Autodesk Inventor part; units mm, degrees
ref_plane "YZ Plane" through (0, 0, 0) normal (1, 0, 0) x (0, 1, 0)
ref_plane "XZ Plane" through (0, 0, 0) normal (0, 1, 0) x (-1, 0, 0)
ref_plane "XY Plane" through (0, 0, 0) normal (0, 0, 1) x (1, 0, 0)
sketch "Sketch1" plane through (0, 0, 0) normal (0, 0, 1) x (1, 0, 0)
  line L0 (-75, -60) -> (75, -60)
  line L1 (75, -60) -> (75, 60)
  line L2 (75, 60) -> (-75, 60)
  line L3 (-75, 60) -> (-75, -60)
  line L4 (-75, -60) -> (75, 60) construction
  line L5 (75, -60) -> (-75, 60) construction
  line L6 (-70, -55) -> (70, -55) construction
  line L7 (70, -55) -> (70, 55) construction
  line L8 (70, 55) -> (-70, 55) construction
  line L9 (-70, 55) -> (-70, -55) construction
  circle A0 centre (-48, 0) radius 15
  circle A1 centre (-55, 55) radius 1.6
  circle A2 centre (-18.3333, 55) radius 1.6
  circle A3 centre (18.3333, 55) radius 1.6
  circle A4 centre (55, 55) radius 1.6
  circle A5 centre (-55.8297, -55) radius 1.6
  circle A6 centre (-19.1631, -55) radius 1.6
  circle A7 centre (17.5036, -55) radius 1.6
  circle A8 centre (54.1703, -55) radius 1.6
  circle A9 centre (-65.3, 4) radius 1.25
  circle A10 centre (-30.7, 4) radius 1.25
  circle A11 centre (-65.3, -40) radius 1.25
  circle A12 centre (-30.7, -40) radius 1.25
  circle A13 centre (48, 0) radius 15
  circle A14 centre (30.7, 4) radius 1.25
  circle A15 centre (65.3, 4) radius 1.25
  circle A16 centre (30.7, -40) radius 1.25
  circle A17 centre (65.3, -40) radius 1.25
  circle A18 centre (0, -25) radius 15
  circle A19 centre (17.3, -29) radius 1.25
  circle A20 centre (-17.3, -29) radius 1.25
  circle A21 centre (17.3, 15) radius 1.25
  circle A22 centre (-17.3, 15) radius 1.25
  line L10 (-62.5, 19) -> (-62.5, 31) construction
  line L11 (-59.5, 19) -> (-59.5, 31) construction
  line L12 (-65.5, 31) -> (-65.5, 19) construction
  arc A23 (-65.5, 19) -> (-59.5, 19) centre (-62.5, 19) ccw construction
  arc A24 (-59.5, 31) -> (-65.5, 31) centre (-62.5, 31) ccw construction
  line L13 (-58, 31) -> (-58, 19)
  arc A25 (-67, 19) -> (-58, 19) centre (-62.5, 19) ccw
  line L14 (-67, 19) -> (-67, 31)
  arc A26 (-58, 31) -> (-67, 31) centre (-62.5, 31) ccw
  line L15 (-12, -44.5) -> (-24, -44.5) construction
  line L16 (-12, -40) -> (-24, -40)
  line L17 (-24, -49) -> (-12, -49)
  arc A27 (-12, -49) -> (-12, -40) centre (-12, -44.5) ccw
  arc A28 (-24, -40) -> (-24, -49) centre (-24, -44.5) ccw
  circle A29 centre (30.7, -18) radius 1.25
  circle A30 centre (65.3, -18) radius 1.25
  circle A31 centre (-65.3, -18) radius 1.25
  circle A32 centre (-30.7, -18) radius 1.25
  circle A33 centre (17.3, -7) radius 1.25
  circle A34 centre (-17.3, -7) radius 1.25
  point P0 (0, 0)
  point P1 (48, 0)
  point P2 (-62.5, 25)
  point P3 (0, 0)
  point P4 (-18, -44.5)
  dimension "d0" = 150
  dimension "d1" = 120
  dimension "d2" = 60
  dimension "d3" = 60
  dimension "d5" = 27
  dimension "d6" = 27
  dimension "d7" = 5
  dimension "d8" = 20
  dimension "d9" = 30
  dimension "d14" = 20
  dimension "d15" = 36.6667
  dimension "d16" = 36.6667
  dimension "d17" = 3.2
  dimension "d18" = 3.2
  dimension "d19" = 3.2
  dimension "d20" = 3.2
  dimension "d21" = 3.2
  dimension "d22" = 3.2
  dimension "d23" = 3.2
  dimension "d24" = 3.2
  dimension "d25" = 4
  dimension "d26" = 17.3
  dimension "d27" = 17.3
  dimension "d28" = 44
  dimension "d29" = 2.5
  dimension "d30" = 2.5
  dimension "d31" = 2.5
  dimension "d32" = 2.5
  dimension "d40" = 40
  dimension "d41" = 30
  dimension "d42" = 4
  dimension "d43" = 17.3
  dimension "d44" = 17.3
  dimension "d45" = 44
  dimension "d46" = 2.5
  dimension "d47" = 2.5
  dimension "d48" = 2.5
  dimension "d49" = 2.5
  dimension "d50" = 40
  dimension "d51" = 30
  dimension "d52" = 4
  dimension "d53" = 17.3
  dimension "d54" = 17.3
  dimension "d55" = 44
  dimension "d56" = 2.5
  dimension "d57" = 2.5
  dimension "d58" = 2.5
  dimension "d59" = 2.5
  dimension "d60" = 40
  dimension "d67" = 6
  dimension "d68" = 6
  dimension "d69" = 12.5
  dimension "d70" = 25
  dimension "d71" = 1.5
  dimension "d80" = 12
  dimension "d81" = 9
  dimension "d82" = 6
  dimension "d83" = 12
  dimension "d86" = 2.5
  dimension "d87" = 2.5
  dimension "d88" = 2.5
  dimension "d89" = 2.5
  dimension "d90" = 22
  dimension "d94" = 2.5
extrude "Extrusion1" add sketch "Sketch1" against normal blind 2 contours L3 L2 L1 L0 | A9 | A10 | A11 | A12 | A14 | A15 | A16 | A17 | A19 | A20 | A21 | A22 | L13 A25 L14 A26 | A27 L17 A28 L16 | A29 | A30 | A31 | A32 | A33 | A34
extrude "Extrusion2" cut sketch "Sketch1" against normal through all contours A9 | A10 | A11 | A12 | A14 | A15 | A16 | A17 | A19 | A20 | A21 | A22 | A29 | A30 | A31 | A32 | A33 | A34
extrude "Extrusion3" cut sketch "Sketch1" against normal blind 10 contours L13 A25 L14 A26
extrude "Extrusion4" cut sketch "Sketch1" against normal through all contours A27 L17 A28 L16
mirror "Mirror1" about plane through (0, 0, 0) normal (1, 0, 0) of "Extrusion3", "Extrusion4"
equation "\"d30\" = d29"
equation "\"d31\" = d29"
equation "\"d47\" = d46"
equation "\"d48\" = d46"
equation "\"d57\" = d56"
equation "\"d58\" = d56"
properties part number "upper plate"
Build history of the part. All positions in model axes, mm. A direction names the side the tool comes from. Give positions to 0.01 mm unless a question says otherwise; leave off trailing zeros. Order: outer loops, then holes, each group sorted by start corner. A loop starts at its lowest first (then second) coordinate and runs counter-clockwise, first axis right, second up. Notation, with made-up numbers: M 70.25,47 L 110.25,47 A13 ccw 110.25,65 Z; hole C -31,-31.5 d11. An arc over 180 degrees is marked long. Use one line per item in the form item = value.
Q1. Slice it at D-D, the plane y = 8.5. Write the cut outline in (x, z), and give its area (3 significant figures).
Conclusion:
outline = M -75,-2 L -60.36,-2 L -60.36,0 L -75,0 Z; M -35.64,-2 L 35.64,-2 L 35.64,0 L -35.64,0 Z; M 60.36,-2 L 75,-2 L 75,0 L 60.36,0 Z
area = 201 mm2
Q2. Slice it at C-C, the plane z = -0.6. State how many separate pieces and enclosed holes the cut face has, and give its area (3 significant figures).
Conclusion:
separate_pieces = 1
enclosed_holes = 33
area = 15,000 mm2
Q3. Pull direction X, two halves, no side cores. Call faces 1 (the flat face through (-1, 1, -2)), 2 (the cylindrical face through (-17.637, -54.519, -0.986)): released by +X, released by -X, zero draft, split by the parting line, or undercut.
Conclusion:
face_1 = zero draft
face_2 = undercut
Q4. Wall check: probe 1 along Y at (x, z) = (-30.7, -0.6); probe 2 along X at (y, z) = (30, -0.85); probe 3 along Y at (x, z) = (-65.5, -1.35). Give the ranges that are in metal, low to high.
Conclusion:
probe_1 = -60 to -41.25, -38.75 to -19.25, -16.75 to 2.75, 5.25 to 60
probe_2 = -75 to -67, -58 to 58, 67 to 75
probe_3 = -60 to -41.23, -38.77 to -19.23, -16.77 to 2.77, 5.23 to 15.65, 34.35 to 60
Q5. Slice it at B-B, the plane x = -48. Write the cut outline in (y, z), and give its area (3 significant figures).
Conclusion:
outline = M -60,-2 L -15,-2 L -15,0 L -60,0 Z; M 15,-2 L 60,-2 L 60,0 L 15,0 Z
area = 180 mm2
Q6. Slice it at A-A, the plane y = -44.5. Write the cut outline in (x, z).
Conclusion:
outline = M -75,-2 L -28.5,-2 L -28.5,0 L -75,0 Z; M -7.5,-2 L 7.5,-2 L 7.5,0 L -7.5,0 Z; M 28.5,-2 L 75,-2 L 75,0 L 28.5,0 Z
Q7. Which spindle directions (+Z, -Z, +X, -X, +Y, -Y) get a long thin tool onto all of the face, cutting with end or side? Do faces 3 (the flat face through (-1, 1, 0)), 4 (the cylindrical face through (-7.5, -44.6, -1)). Say none if no direction does.
Conclusion:
face_3 = +Z, +X, -X, +Y, -Y
face_4 = +Z, -Z
